from build123d import *

# Parameters (mm, degrees)
F0_W     = 20
F0_H     = 20
F0_W_2   = 19
F0_H_2   = 19
F1_DEPTH = 105
F2_R     = 1.5
F3_DEPTH = 25


with BuildPart() as f1:
    # F0 (on Top) → F1 (new body)
    with BuildSketch(Plane.XY):
        Rectangle(F0_W, F0_H)
        Rectangle(F0_W_2, F0_H_2, mode=Mode.SUBTRACT)
    extrude(amount=F1_DEPTH)

    # F2 (on face) → F3 (cut)
    with BuildSketch(Plane(origin=(0, 10, 0), x_dir=(-1, 0, 0), z_dir=(0, 1, 0))):
        with Locations((0, 90)):
            Circle(F2_R)
        with Locations((0, 75)):
            Circle(F2_R)
        with Locations((0, 60)):
            Circle(F2_R)
        with Locations((0, 45)):
            Circle(F2_R)
        with Locations((0, 30)):
            Circle(F2_R)
        with Locations((0, 15)):
            Circle(F2_R)
    extrude(amount=-F3_DEPTH, mode=Mode.SUBTRACT)


solid = f1.part
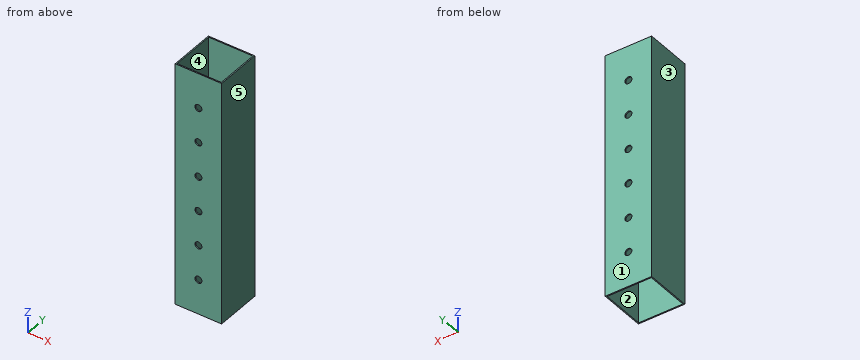
CAD build for the part. Positions are in the model's coordinates, mm. Face numbers are marked on the shaded views. A direction names the side the tool comes from. Coordinates: 2 decimals unless noted, no trailing zeros. Write each loop counter-clockwise with the first axis right and the second up, starting at its lowest first coordinate (ties: lowest second). Pieces come first, ordered by that corner, then holes. Notation, with made-up numbers: M -18.75,1.25 L 9.25,1.25 A13 ccw 9.25,26.25 Z; hole C 28,77.5 d7. An arc over 180 degrees is marked long. Return JSON: item names as keys, results as strings.
Item 1: Which spindle directions (+Z, -Z, +X, -X, +Y, -Y) get a long thin tool onto all of the face, cutting with end or side? Do the marked faces 4 and 5. Say none if no direction does.
Findings below:
{"face 4": "+Z, -Z", "face 5": "+Z, -Z, +X, +Y, -Y"}
Item 2: Two-plate mould, pull along Y, no slides. Class the marked faces 1, 2 and 3: +Y half, -Y half, draft (parallel to the pull), parting line (faces both ways), or undercut.
Findings below:
{"face 1": "+Y half", "face 2": "undercut", "face 3": "draft"}
Item 3: Slice it at C-C, the plane z = 60. Write the cut outline in (x, y), and give its area (3 significant figures).
Findings below:
{"outline": "M -10,-10 L -1.5,-10 L -1.5,-9.5 L -9.5,-9.5 L -9.5,9.5 L -1.5,9.5 L -1.5,10 L -10,10 Z; M 1.5,-10 L 10,-10 L 10,10 L 1.5,10 L 1.5,9.5 L 9.5,9.5 L 9.5,-9.5 L 1.5,-9.5 Z", "area": "36.0 mm2"}
Item 4: Slice it at A-A, the plane z = 87. Write the cut outline in (x, y).
Findings below:
{"outline": "M -10,-10 L 10,-10 L 10,10 L -10,10 Z; hole M -9.5,-9.5 L 9.5,-9.5 L 9.5,9.5 L -9.5,9.5 Z"}
Item 5: Drop flat-ended pins along their axis: pin 1 Ø2.5 at (x, z) = (0, 60) entering from -Y; pin 2 Ø3.5 at (x, z) = (0, 30) entering from +Y. Give the stop position or say it passes through.
Findings below:
{"pin 1": "passes through", "pin 2": "stops at y = 10"}
Item 6: Slice it at B-B, the plane x = -3.75. Write the cut outline in (y, z).
Findings below:
{"outline": "M -10,0 L -9.5,0 L -9.5,105 L -10,105 Z; M 9.5,0 L 10,0 L 10,105 L 9.5,105 Z"}
Item 7: Probe line 1 (X direction, y = -3.5, z = 81); line 2 (X direction, y = -9.9, z = 75). List the from-to ranges inside material, lowest first. Write a range as from..to.
Findings below:
{"line 1": "x = -10..-9.5, 9.5..10", "line 2": "x = -10..-1.5, 1.5..10"}
